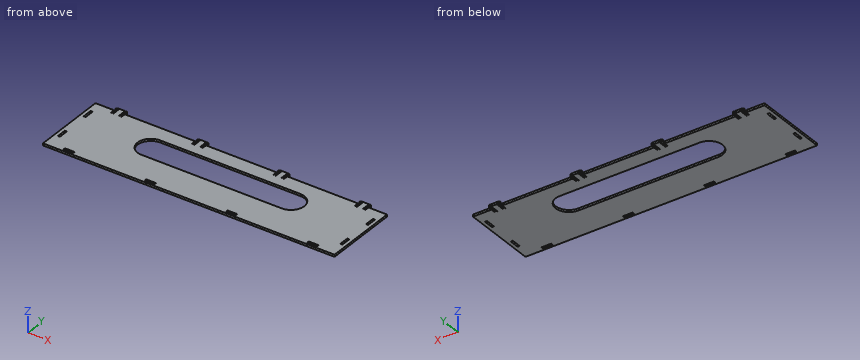
from build123d import *

# Parameters (mm, degrees)
BOSS_EXTRUDE1_DEPTH = 3
CUT_EXTRUDE2_DEPTH  = 4
SKETCH8_W           = 14
SKETCH8_H           = 3
CUT_EXTRUDE3_DEPTH  = 3
SKETCH9_W           = 3
SKETCH9_H           = 14
CUT_EXTRUDE4_DEPTH  = 3


with BuildPart() as part:
    # Sketch1 → Boss-Extrude1 (new body)
    with BuildSketch(Plane.XY):
        Polygon((208, 50), (182, 50), (181.5, 42.997828908), (181, 42.997828908), (181, 51.997828908), (181.5, 52.997828908), (182, 53.497828908), (182, 54.497828908), (180.5, 55.997828908), (179, 55.997828908), (178.5, 42.997828908), (178, 42.997828908), (178, 55.997828908), (170, 55.997828908), (170, 42.997828908), (169.5, 42.997828908), (169, 55.997828908), (167.5, 55.997828908), (166, 54.497828908), (166, 53.497828908), (166.5, 52.997828908), (167, 51.997828908), (167, 42.997828908), (166.5, 42.997828908), (166, 50), (66, 50), (65.5, 42.997828908), (65, 42.997828908), (65, 51.997828908), (65.5, 52.997828908), (66, 53.497828908), (66, 54.497828908), (64.5, 55.997828908), (63, 55.997828908), (62.5, 42.997828908), (62, 42.997828908), (62, 55.997828908), (54, 55.997828908), (54, 42.997828908), (53.5, 42.997828908), (53, 55.997828908), (51.5, 55.997828908), (50, 54.497828908), (50, 53.497828908), (50.5, 52.997828908), (51, 51.997828908), (51, 42.997828908), (50.5, 42.997828908), (50, 50), (-50, 50), (-50.5, 42.997828908), (-51, 42.997828908), (-51, 51.997828908), (-50.5, 52.997828908), (-50, 53.497828908), (-50, 54.497828908), (-51.5, 55.997828908), (-53, 55.997828908), (-53.5, 42.997828908), (-54, 42.997828908), (-54, 55.997828908), (-62, 55.997828908), (-62, 42.997828908), (-62.5, 42.997828908), (-63, 55.997828908), (-64.5, 55.997828908), (-66, 54.497828908), (-66, 53.497828908), (-65.5, 52.997828908), (-65, 51.997828908), (-65, 42.997828908), (-65.5, 42.997828908), (-66, 50), (-166, 50), (-166.5, 42.997828908), (-167, 42.997828908), (-167, 51.997828908), (-166.5, 52.997828908), (-166, 53.497828908), (-166, 54.497828908), (-167.5, 55.997828908), (-169, 55.997828908), (-169.5, 42.997828908), (-170, 42.997828908), (-170, 55.997828908), (-178, 55.997828908), (-178, 42.997828908), (-178.5, 42.997828908), (-179, 55.997828908), (-180.5, 55.997828908), (-182, 54.497828908), (-182, 53.497828908), (-181.5, 52.997828908), (-181, 51.997828908), (-181, 42.997828908), (-181.5, 42.997828908), (-182, 50), (-208, 50), (-208, -56), (208, -56), align=None)
    extrude(amount=BOSS_EXTRUDE1_DEPTH)

    # Sketch4 → Cut-Extrude2 (cut, through all)
    with BuildSketch(Plane.XY.offset(3)):
        with BuildLine():
            Line((-100, 28), (100, 28))
            ThreePointArc((100, 28), (119, 9), (100, -10))
            Line((100, -10), (-100, -10))
            ThreePointArc((-100, -10), (-119, 9), (-100, 28))
        make_face()
    extrude(amount=-CUT_EXTRUDE2_DEPTH, mode=Mode.SUBTRACT)

    # Sketch8 → Cut-Extrude3 (cut)
    with BuildSketch(Plane.XY.offset(3)):
        with Locations((174, -51.5)):
            Rectangle(SKETCH8_W, SKETCH8_H)
        with Locations((-174, -51.5)):
            Rectangle(SKETCH8_W, SKETCH8_H)
        with Locations((58, -51.5)):
            Rectangle(SKETCH8_W, SKETCH8_H)
        with Locations((-58, -51.5)):
            Rectangle(SKETCH8_W, SKETCH8_H)
    extrude(amount=-CUT_EXTRUDE3_DEPTH, mode=Mode.SUBTRACT)

    # Sketch9 → Cut-Extrude4 (cut)
    with BuildSketch(Plane.XY.offset(3)):
        with Locations((201.5, 26)):
            Rectangle(SKETCH9_W, SKETCH9_H)
        with Locations((-201.5, 26)):
            Rectangle(SKETCH9_W, SKETCH9_H)
        with Locations((-201.5, -26)):
            Rectangle(SKETCH9_W, SKETCH9_H)
        with Locations((201.5, -26)):
            Rectangle(SKETCH9_W, SKETCH9_H)
    extrude(amount=-CUT_EXTRUDE4_DEPTH, mode=Mode.SUBTRACT)


solid = part.part
For this review, take the finished solid that the model builds, in its own axes (mm). Round coordinates to 2 decimals unless told otherwise and drop trailing zeros. Loops run counter-clockwise (first coordinate to the right, second up) from the corner with the lowest first, then second, coordinate; pieces in that order, holes last. Notation, with made-up numbers: (-8.75, 42) - (38.25, 42) arc R19 ccw to (38.25, 68) - close; hole circle Ø5 at (64.25, -11.75). An arc over 180 degrees is marked (long way). One line per question, with ' | ' between items.
Q1. Take a section at B-B (y = 9). Give the boundary of the cut face in (x, z), and give its area (3 significant figures).
Taken from the geometry:
outline: (-208, 0) - (-119, 0) - (-119, 3) - (-208, 3) - close; (119, 0) - (208, 0) - (208, 3) - (119, 3) - close | area: 534 mm²
Q2. Take a section at C-C (x = 140). Give the boundary of the cut face in (y, z), and give its area (3 significant figures).
Taken from the geometry:
outline: (-56, 0) - (50, 0) - (50, 3) - (-56, 3) - close | area: 318 mm²
Q3. For pin 1 (0.9 mm diameter, centred on y = 51, z = 1, fed in from +X); pin 2 (1.5 mm diameter, centred on x = 8, z = 1.5, fed in from +Y); pin 3 (1.1 mm diameter, centred on y = 54, z = 1.5, fed in from +X), all flat-tipped, find the tip position at first contact; note any pin that passes through.
Taken from the geometry:
pin 1: stops at x = 181 | pin 2: stops at y = 50 | pin 3: stops at x = 182
Q4. For line 1 along Y through (x, z) = (77, 1.8); line 2 along Y through (x, z) = (-186, 0.85); line 3 along Y through (x, z) = (115, 1.6), list the stretches that pass through material, from the lowest coordinate up. Write a range as [from, to].
Taken from the geometry:
line 1: y = [-56, -10], [28, 50] | line 2: y = [-56, 50] | line 3: y = [-56, -2.66], [20.66, 50]
Q5. Take a section at D-D (z = 1.2). State how many separate pieces and enclosed holes the cut face has, and give its area (3 significant figures).
Taken from the geometry:
separate pieces: 1 | enclosed holes: 9 | area: 35,300 mm²
Q6. Take a section at A-A (x = 44.5). Give the boundary of the cut face in (y, z).
Taken from the geometry:
outline: (-56, 0) - (-10, 0) - (-10, 3) - (-56, 3) - close; (28, 0) - (50, 0) - (50, 3) - (28, 3) - close
